```python
from build123d import *

# Parameters (mm, degrees)
SKETCH1_R           = 2.54
SKETCH1_R_2         = 14.2875
BOSS_EXTRUDE1_DEPTH = 6.35
SKETCH3_R           = 175
CUT_EXTRUDE1_DEPTH  = 7.35
FILLET1_R           = 2.54


with BuildPart() as part:
    # Sketch1 → Boss-Extrude1 (new body)
    with BuildSketch(Plane(origin=(0, 0, 0), x_dir=(1, 0, 0), z_dir=(0, 1, 0))):
        with BuildLine():
            Line((-10.301536111, 44.922263418), (-42.486128255, 37.541719497))
            ThreePointArc((-42.486128255, 37.541719497), (-48.376257791, 32.787738977), (-48.258608454, 25.219376184))
            Line((-48.258608454, 25.219376184), (-30.922632743, -8.978011563))
            ThreePointArc((-30.922632743, -8.978011563), (-29.753188396, -10.670651305), (-28.173552503, -11.988748349))
            Line((-28.173552503, -11.988748349), (1.485082186, -30.582244497))
            ThreePointArc((1.485082186, -30.582244497), (3.286793362, -31.407609936), (5.240405543, -31.740462332))
            Line((5.240405543, -31.740462332), (43.718670442, -33.216869907))
            ThreePointArc((43.718670442, -33.216869907), (50.700017874, -30.096753296), (52.467298047, -22.656923969))
            Line((52.467298047, -22.656923969), (45.086754126, 9.527668174))
            ThreePointArc((45.086754126, 9.527668174), (41.870070274, 14.491711544), (36.213465331, 16.221336388))
            Line((36.213465331, 16.221336388), (24.402688291, 15.597131936))
            ThreePointArc((24.402688291, 15.597131936), (22.820864626, 15.76285886), (21.367816063, 16.409605637))
            Line((21.367816063, 16.409605637), (5.906875614, 26.450057762))
            ThreePointArc((5.906875614, 26.450057762), (4.742385284, 27.493110687), (3.950204921, 28.84086712))
            Line((3.950204921, 28.84086712), (-0.341397124, 39.683137821))
            ThreePointArc((-0.341397124, 39.683137821), (-4.350888408, 44.147873767), (-10.301536111, 44.922263418))
        make_face()
        with Locations((-5.53256927, 24.126065418)):
            Circle(SKETCH1_R, mode=Mode.SUBTRACT)
        with Locations((24.290556126, 4.758701333)):
            Circle(SKETCH1_R, mode=Mode.SUBTRACT)
        with Locations((5.53256927, -24.126065418)):
            Circle(SKETCH1_R, mode=Mode.SUBTRACT)
        with Locations((-24.126065418, -5.53256927)):
            Circle(SKETCH1_R, mode=Mode.SUBTRACT)
        Circle(SKETCH1_R_2, mode=Mode.SUBTRACT)
        with BuildLine():
            Line((40.135278412, 8.392199879), (47.515822333, -23.792392264))
            ThreePointArc((47.515822333, -23.792392264), (44.84461714, -28.053253071), (40.583756333, -25.382047878))
            Line((40.583756333, -25.382047878), (33.203212412, 6.802544265))
            ThreePointArc((33.203212412, 6.802544265), (35.874417605, 11.063405072), (40.135278412, 8.392199879))
        make_face(mode=Mode.SUBTRACT)
        with BuildLine():
            Line((-7.576412202, 33.038721704), (-39.761004345, 25.658177783))
            ThreePointArc((-39.761004345, 25.658177783), (-44.021865152, 28.329382976), (-41.350659959, 32.590243783))
            Line((-41.350659959, 32.590243783), (-9.166067816, 39.970787704))
            ThreePointArc((-9.166067816, 39.970787704), (-4.905207009, 37.299582511), (-7.576412202, 33.038721704))
        make_face(mode=Mode.SUBTRACT)
    extrude(amount=BOSS_EXTRUDE1_DEPTH)

    # Sketch3 → Cut-Extrude1 (cut, through all)
    with BuildSketch(Plane(origin=(0, 6.35, 0), x_dir=(1, 0, 0), z_dir=(0, 1, 0))):
        with Locations((111.500681804, 171.695993352)):
            Circle(SKETCH3_R)
        with BuildLine():
            Line((29.692484449, -0.615642385), (35.632280619, -26.517516174))
            ThreePointArc((35.632280619, -26.517516174), (35.636280873, -26.534877998), (35.640316938, -26.552231532))
            Line((35.640316938, -26.552231532), (12.991771922, -25.68320889))
            ThreePointArc((12.991771922, -25.68320889), (12.360044144, -20.742282498), (8.810828705, -17.247299898))
            ThreePointArc((8.810828705, -17.247299898), (16.242952225, -10.548296511), (19.339879369, -1.033983679))
            ThreePointArc((19.339879369, -1.033983679), (24.598223728, -2.85508489), (29.692484449, -0.615642385))
        make_face()
        with BuildLine():
            Line((-38.62553605, 20.706702069), (-12.723662261, 26.646498238))
            ThreePointArc((-12.723662261, 26.646498238), (-12.567344847, 21.197527799), (-8.810828705, 17.247299898))
            ThreePointArc((-8.810828705, 17.247299898), (-16.40945516, 10.287363006), (-19.363045216, 0.415374791))
            ThreePointArc((-19.363045216, 0.415374791), (-23.979054852, 2.086012481), (-28.656078555, 0.594696105))
            Line((-28.656078555, 0.594696105), (-38.829256345, 20.662566027))
            ThreePointArc((-38.829256345, 20.662566027), (-38.727263029, 20.684019377), (-38.62553605, 20.706702069))
        make_face()
    extrude(amount=-CUT_EXTRUDE1_DEPTH, mode=Mode.SUBTRACT)

    # Fillet1
    fillet1_edges = [part.edges().sort_by_distance(p)[0] for p in [
        (35.640316938, 3.175, 26.552231532),
        (8.810828705, 3.175, 17.247299898),
        (12.991771922, 3.175, 25.68320889),
        (29.692484449, 3.175, 0.615642385),
        (19.339879369, 3.175, 1.033983679),
        (-38.829256345, 3.175, -20.662566027),
        (-28.656078555, 3.175, -0.594696105),
        (-19.363045216, 3.175, -0.415374791),
        (-8.810828705, 3.175, -17.247299898),
        (-12.723662261, 3.175, -26.646498238),
    ]]
    fillet(fillet1_edges, radius=FILLET1_R)


solid = part.part
```
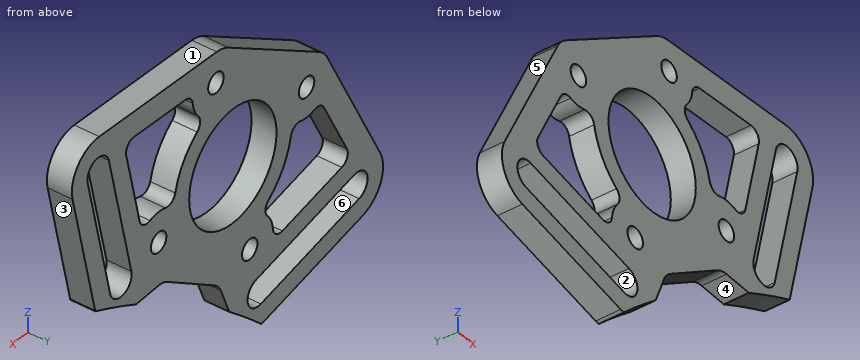
Here's how the part is built. I have some questions about the finished solid (model axes, mm). Face numbers are marked on the shaded views. A direction names the side the tool comes from. Round coordinates to 2 decimals unless told otherwise and drop trailing zeros. Order: outer loops, then holes, each group sorted by start corner. A loop starts at its lowest first (then second) coordinate and runs counter-clockwise, first axis right, second up. Notation, with made-up numbers: M 39,35 L 75,35 A18 ccw 75,67 Z; hole C 1.25,65.25 d1. An arc over 180 degrees is marked long. Use CSV: the item, a comma, the result in double quotes.
1) I want a section at B-B (z = 0). List the corners of the cut face in (x, y) for me, then the cut area to 3 significant figures.
Taken from the geometry:
outline,"M -35.47,0 L -14.29,0 L -14.29,6.35 L -35.47,6.35 Z; M 14.29,0 L 34.76,0 L 34.76,6.35 L 14.29,6.35 Z; M 42.06,0 L 47.27,0 L 47.27,6.35 L 42.06,6.35 Z"
area,"298 mm^2"
2) I'm going to push flat-ended pins straight in: P1, Ø4.5, axis at x = 24.29, z = -4.76, coming from the +Y side; P2, Ø1.5, axis at x = -3, y = 5.5, coming from the +Z side; P3, Ø1, axis at x = -16.5, y = 2.5, coming from the +Z side; P4, Ø2, axis at y = 5, z = 14, coming from the -X side. Where does each tip first touch, or does it pass through?
Taken from the geometry:
P1,"through"
P2,"z = 28.24"
P3,"z = 19.62"
P4,"x = -26.56"
3) I want a section at A-A (x = 37). List the corners of the cut face in (y, z) for me.
Taken from the geometry:
outline,"M 0,-13.35 L 6.35,-13.35 L 6.35,-11.14 L 0,-11.14 Z; M 0,9.75 L 6.35,9.75 L 6.35,32.96 L 0,32.96 Z"
4) I want a section at C-C (x = 0). List the corners of the cut face in (y, z) for me, then the cut area to 3 significant figures.
Taken from the geometry:
outline,"M 0,-36.82 L 6.35,-36.82 L 6.35,-14.29 L 0,-14.29 Z; M 0,14.29 L 6.35,14.29 L 6.35,29.65 L 0,29.65 Z"
area,"241 mm^2"
5) I want a section at D-D (y = 2.5). Count the separate pieces of the cut face and the enclosed holes in it, then the cut area to 3 significant figures.
Taken from the geometry:
separate pieces,"1"
enclosed holes,"9"
area,"2,810 mm^2"
6) I need wall thicknesses on line 1 along X through (y, z) = (5, 0); line 2 along Z through (x, y) = (-31, 1.75); line 3 along X through (y, z) = (2, 16.5). Which ranges of each line are inside material? Lowest first, please. Write a range as [from, to].
Taken from the geometry:
line 1,"[-35.47, -14.29], [14.29, 34.76], [42.06, 47.27]"
line 2,"[-40.18, -34.96], [-27.67, -22.46], [-5.22, 8.83]"
line 3,"[-20.98, 10.87], [33.34, 38.55], [45.84, 51.06]"
7) On a 3-axis mill with a long thin cutter (end or side, diameter ignored), from which of +Z, -Z, +X, -X, +Y, -Y can I reach the whole of each face in a straight line? I mean the marked faces 4, 5 and 6. Say none if no direction works.
Taken from the geometry:
face 4,"-Z, +Y, -Y"
face 5,"+Z, -X, +Y, -Y"
face 6,"+Y, -Y"
8) If we mould it in two halves opening along X, with no side actions, what happens to the marked faces 1, 2 and 3? For each: pulls with the +X half, pulls with the -X half, needs draft (parallel to the pull), parting line crosses it, or undercut.
Taken from the geometry:
face 1,"pulls with the -X half"
face 2,"undercut"
face 3,"pulls with the +X half"
